Read the model definition and answer for the solid it produces. Units are mm, in the model's axes. Face numbers are marked on the shaded views. A direction names the side the tool comes from. Coordinates: 2 decimals unless noted, no trailing zeros. Write each loop counter-clockwise with the first axis right and the second up, starting at its lowest first coordinate (ties: lowest second). Pieces come first, ordered by that corner, then holes. Notation, with made-up numbers: (70, 37.25) -> (121, 37.25) arc R11 cw to (121, 44.25) -> close; hole circle Ø9 at (-27, 27). An arc over 180 degrees is marked (long way). Answer in a Markdown table with one row per item. Add a question column.
Item 1: Section B-B on y = 31 is taken. Count the separate pieces of the cut face and the enclosed holes in it, then the cut area to 3 significant figures.
Item 2: Straight lines are drawn through the part: line 1 (X direction, y = 26, z = -29.5); line 2 (Y direction, x = -16, z = 1); line 3 (X direction, y = 12.5, z = 24). For each, find the intervals that lie inside material, in ascending order. Write a range as from..to.
Item 3: Given pin 1 Ø3 at (x, z) = (-44.9, -30) entering from +Y; pin 2 Ø2.5 at (x, y) = (34.5, 3.5) entering from -Z; pin 3 Ø2.5 at (y, z) = (20, 49.5) entering from -X; pin 4 Ø2.5 at (y, z) = (25, -48) entering from -X, each flat-ended and moving along its own axis, determine where each tip first touches the part or whether it passes through.
Item 4: Which of the six approach directions +Z, -Z, +X, -X, +Y, -Y give full straight-line access (tool end or side, diameter ignored) to the marked faces 1, 2 and 3?
Item 5: For a pull along Z with two mould halves and no side action, classify the marked faces 4, 5, 6 and 7 as +Z half, -Z half, draft (parallel to the pull), parting line (faces both ways), or undercut.
Item 6: Section A-A on x = 0 is taken. Write down the section's boundary in (y, z).
Item 7: Section C-C on z = 0 is taken. Write down the section's boundary in (x, y), then the cut area to 3 significant figures.
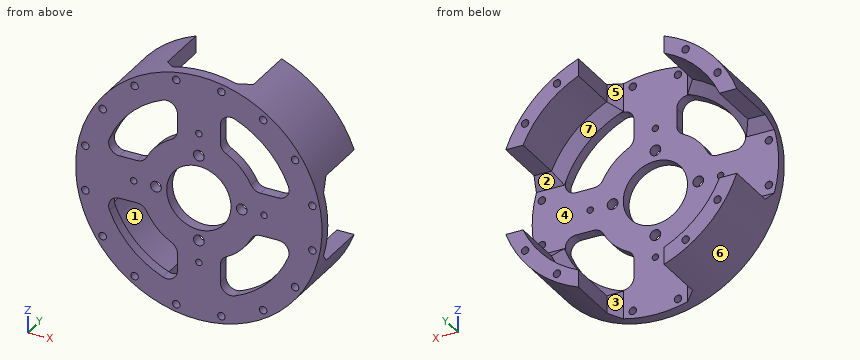
```python
from build123d import *

# Parameters (mm, degrees)
SKETCH1_R           = 57.5
BOSS_EXTRUDE1_DEPTH = 34.6
SKETCH2_R           = 50
CUT_EXTRUDE1_DEPTH  = 29.6
SKETCH3_R           = 2.5
SKETCH3_R_2         = 15
CUT_EXTRUDE2_DEPTH  = 31.8
SKETCH4_R           = 1.5
SKETCH4_R_2         = 1.75
CUT_EXTRUDE3_DEPTH  = 50
SKETCH9_W           = 40
SKETCH9_H           = 29.6
CUT_EXTRUDE4_DEPTH  = 72
CIRPATTERN1_COUNT   = 4
FILLET2_R           = 5
CHAMFER1_SIZE       = 5


with BuildPart() as part:
    # Sketch1 → Boss-Extrude1 (new body)
    with BuildSketch(Plane(origin=(0, 0, 0), x_dir=(1, 0, 0), z_dir=(0, 1, 0))):
        with Locations(Location((0, 0, 0), (0, 0, 270))):
            Circle(SKETCH1_R)
    extrude(amount=BOSS_EXTRUDE1_DEPTH)

    # Sketch2 → Cut-Extrude1 (cut)
    with BuildSketch(Plane(origin=(0, 34.6, 0), x_dir=(1, 0, 0), z_dir=(0, 1, 0))):
        with Locations(Location((0, 0, 0), (0, 0, 270))):
            Circle(SKETCH2_R)
    extrude(amount=-CUT_EXTRUDE1_DEPTH, mode=Mode.SUBTRACT)

    # Sketch3 → Cut-Extrude2 (cut)
    with BuildSketch(Plane.XZ):
        with BuildLine():
            Line((-10, 25.617376915), (-10, 43.874821937))
            ThreePointArc((-10, 43.874821937), (-31.819805153, 31.819805153), (-43.874821937, 10))
            Line((-43.874821937, 10), (-25.617376915, 10))
            ThreePointArc((-25.617376915, 10), (-19.445436483, 19.445436483), (-10, 25.617376915))
        make_face()
        with BuildLine():
            Line((25.617376915, 10), (43.874821937, 10))
            ThreePointArc((43.874821937, 10), (31.819805153, 31.819805153), (10, 43.874821937))
            Line((10, 43.874821937), (10, 25.617376915))
            ThreePointArc((10, 25.617376915), (19.445436483, 19.445436483), (25.617376915, 10))
        make_face()
        with BuildLine():
            ThreePointArc((10, -43.874821937), (31.819805153, -31.819805153), (43.874821937, -10))
            Line((43.874821937, -10), (25.617376915, -10))
            ThreePointArc((25.617376915, -10), (19.445436483, -19.445436483), (10, -25.617376915))
            Line((10, -25.617376915), (10, -43.874821937))
        make_face()
        with BuildLine():
            ThreePointArc((-43.874821937, -10), (-31.819805153, -31.819805153), (-10, -43.874821937))
            Line((-10, -43.874821937), (-10, -25.617376915))
            ThreePointArc((-10, -25.617376915), (-19.445436483, -19.445436483), (-25.617376915, -10))
            Line((-25.617376915, -10), (-43.874821937, -10))
        make_face()
        with Locations(Location((-20, 0, 0), (0, 0, 270))):
            Circle(SKETCH3_R)
        with Locations(Location((0, 0, 0), (0, 0, 270))):
            Circle(SKETCH3_R_2)
        with Locations(Location((0, 20, 0), (0, 0, 270))):
            Circle(SKETCH3_R)
        with Locations(Location((20, 0, 0), (0, 0, 270))):
            Circle(SKETCH3_R)
        with Locations(Location((0, -20, 0), (0, 0, 270))):
            Circle(SKETCH3_R)
    extrude(amount=-CUT_EXTRUDE2_DEPTH, mode=Mode.SUBTRACT)

    # Sketch4 → Cut-Extrude3 (cut)
    with BuildSketch(Plane.XZ):
        with Locations(Location((0, 30.405591591, 0), (0, 0, 270))):
            Circle(SKETCH4_R)
        with Locations(Location((30.405591591, 0, 0), (0, 0, 270))):
            Circle(SKETCH4_R)
        with Locations(Location((0, -30.405591591, 0), (0, 0, 270))):
            Circle(SKETCH4_R)
        with Locations(Location((-30.405591591, 0, 0), (0, 0, 270))):
            Circle(SKETCH4_R)
        with Locations(Location((-10.534877389, 52.962405142, 0), (0, 0, 270))):
            Circle(SKETCH4_R_2)
        with Locations(Location((10.534877389, 52.962405142, 0), (0, 0, 270))):
            Circle(SKETCH4_R_2)
        with Locations(Location((30.000792583, 44.899359064, 0), (0, 0, 270))):
            Circle(SKETCH4_R_2)
        with Locations(Location((44.899359064, 30.000792583, 0), (0, 0, 270))):
            Circle(SKETCH4_R_2)
        with Locations(Location((52.962405142, 10.534877389, 0), (0, 0, 270))):
            Circle(SKETCH4_R_2)
        with Locations(Location((52.962405142, -10.534877389, 0), (0, 0, 270))):
            Circle(SKETCH4_R_2)
        with Locations(Location((44.899359064, -30.000792583, 0), (0, 0, 270))):
            Circle(SKETCH4_R_2)
        with Locations(Location((30.000792583, -44.899359064, 0), (0, 0, 270))):
            Circle(SKETCH4_R_2)
        with Locations(Location((10.534877389, -52.962405142, 0), (0, 0, 270))):
            Circle(SKETCH4_R_2)
        with Locations(Location((-10.534877389, -52.962405142, 0), (0, 0, 270))):
            Circle(SKETCH4_R_2)
        with Locations(Location((-30.000792583, -44.899359064, 0), (0, 0, 270))):
            Circle(SKETCH4_R_2)
        with Locations(Location((-44.899359064, -30.000792583, 0), (0, 0, 270))):
            Circle(SKETCH4_R_2)
        with Locations(Location((-52.962405142, -10.534877389, 0), (0, 0, 270))):
            Circle(SKETCH4_R_2)
        with Locations(Location((-52.962405142, 10.534877389, 0), (0, 0, 270))):
            Circle(SKETCH4_R_2)
        with Locations(Location((-44.899359064, 30.000792583, 0), (0, 0, 270))):
            Circle(SKETCH4_R_2)
        with Locations(Location((-30.000792583, 44.899359064, 0), (0, 0, 270))):
            Circle(SKETCH4_R_2)
    extrude(amount=-CUT_EXTRUDE3_DEPTH, mode=Mode.SUBTRACT)

    # Sketch9 → Cut-Extrude4 (cut)
    with BuildSketch(Plane.XY):
        with Locations((0, 19.8)):
            Rectangle(SKETCH9_W, SKETCH9_H)
    cut_extrude4 = extrude(amount=-CUT_EXTRUDE4_DEPTH, mode=Mode.SUBTRACT)

    # CirPattern1: Cut-Extrude4 ×4 about axis
    cirpattern1_axis = Axis((0, 0, 0), (0, 1, 0))
    for i in range(1, CIRPATTERN1_COUNT):
        add(cut_extrude4.rotate(cirpattern1_axis, i * 360 / CIRPATTERN1_COUNT), mode=Mode.SUBTRACT)

    # Fillet2
    fillet2_edges = [part.edges().sort_by_distance(p)[0] for p in [
        (43.874821937, 2.5, 10),
        (25.617376915, 2.5, 10),
        (10, 2.5, 25.617376915),
        (10, 2.5, 43.874821937),
        (10, 2.5, -43.874821937),
        (10, 2.5, -25.617376915),
        (25.617376915, 2.5, -10),
        (43.874821937, 2.5, -10),
        (-43.874821937, 2.5, -10),
        (-25.617376915, 2.5, -10),
        (-10, 2.5, -25.617376915),
        (-10, 2.5, -43.874821937),
        (-10, 2.5, 43.874821937),
        (-10, 2.5, 25.617376915),
        (-25.617376915, 2.5, 10),
        (-43.874821937, 2.5, 10),
    ]]
    fillet(fillet2_edges, radius=FILLET2_R)

    # Chamfer1
    chamfer1_edges = [part.edges().sort_by_distance(p)[0] for p in [
        (-35.355339059, 5, -35.355339059),
        (-20, 5, -49.867701791),
        (20, 5, -49.867701791),
        (-35.355339059, 5, 35.355339059),
        (35.355339059, 5, 35.355339059),
        (35.355339059, 5, -35.355339059),
        (-49.867701791, 5, 20),
        (20, 5, 49.867701791),
        (49.867701791, 5, -20),
        (49.867701791, 5, 20),
        (-20, 5, 49.867701791),
        (-49.867701791, 5, -20),
    ]]
    chamfer(chamfer1_edges, length=CHAMFER1_SIZE - 0.0001)  # a hair under: the kernel refuses the full size


solid = part.part
```
Results below:
| question | item | result |
|---|---|---|
| 1 | separate pieces | 4 |
| 1 | enclosed holes | 8 |
| 1 | area | 1,230 mm2 |
| 2 | line 1 | x = -49.36..-46.58, -43.22..-40.37, 40.37..43.22, 46.58..49.36 |
| 2 | line 2 | y = 0..5 |
| 2 | line 3 | x = -52.25..-43.86, 43.86..52.25 |
| 3 | pin 1 | passes through |
| 3 | pin 2 | stops at z = -46.91 |
| 3 | pin 3 | stops at x = -31.28 |
| 3 | pin 4 | stops at x = -33.48 |
| 4 | face 1 | +Y |
| 4 | face 2 | +X, -X, +Y |
| 4 | face 3 | +Z, -Z, +Y |
| 5 | face 4 | undercut |
| 5 | face 5 | draft |
| 5 | face 6 | parting line |
| 5 | face 7 | undercut |
| 6 | outline | (0, -57.5) -> (5, -57.5) -> (5, -31.91) -> (0, -31.91) -> close; (0, -28.91) -> (5, -28.91) -> (5, -22.5) -> (0, -22.5) -> close; (0, -17.5) -> (5, -17.5) -> (5, -15) -> (0, -15) -> close; (0, 15) -> (5, 15) -> (5, 17.5) -> (0, 17.5) -> close; (0, 22.5) -> (5, 22.5) -> (5, 28.91) -> (0, 28.91) -> close; (0, 31.91) -> (5, 31.91) -> (5, 57.5) -> (0, 57.5) -> close |
| 7 | outline | (-57.5, 0) -> (-31.91, 0) -> (-31.91, 5) -> (-57.5, 5) -> close; (-28.91, 0) -> (-22.5, 0) -> (-22.5, 5) -> (-28.91, 5) -> close; (-17.5, 0) -> (-15, 0) -> (-15, 5) -> (-17.5, 5) -> close; (15, 0) -> (17.5, 0) -> (17.5, 5) -> (15, 5) -> close; (22.5, 0) -> (28.91, 0) -> (28.91, 5) -> (22.5, 5) -> close; (31.91, 0) -> (57.5, 0) -> (57.5, 5) -> (31.91, 5) -> close |
| 7 | area | 345 mm2 |
